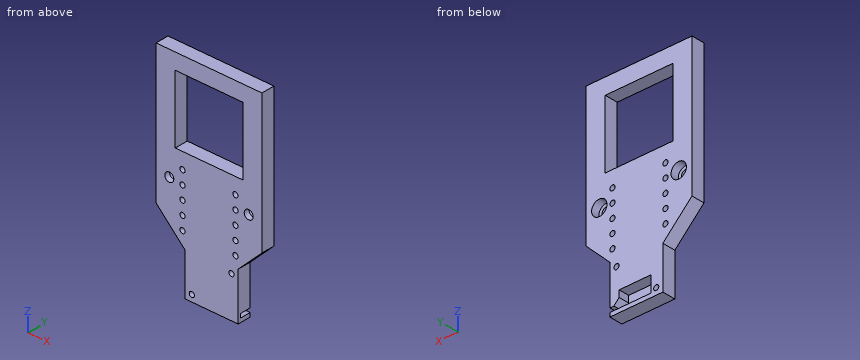
from build123d import *

# Parameters (mm, degrees)
SKETCH1_W           = 40
SKETCH1_H           = 45
SKETCH1_R           = 1.7
BOSS_EXTRUDE1_DEPTH = 5
SKETCH7_R           = 2.9
CUT_EXTRUDE6_DEPTH  = 3
SKETCH4_R           = 0.975
CUT_EXTRUDE3_DEPTH  = 31.516389039
SKETCH5_R           = 0.975
CUT_EXTRUDE4_DEPTH  = 31.516389039
LPATTERN1_COUNT     = 5
LPATTERN1_PITCH     = 5
CUT_EXTRUDE7_DEPTH  = 4
FILLET2_R           = 3
CHAMFER2_SIZE       = 2
CUT_EXTRUDE8_DEPTH  = 31.516389039
SKETCH10_W          = 40
SKETCH10_H          = 34.5
SKETCH10_W_2        = 25.5
SKETCH10_H_2        = 25.5
BOSS_EXTRUDE2_DEPTH = 5


with BuildPart() as part:
    # Sketch1 → Boss-Extrude1 (new body)
    with BuildSketch(Plane(origin=(0, 0, 0), x_dir=(1, 0, 0), z_dir=(0, 1, 0))):
        Rectangle(SKETCH1_W, SKETCH1_H)
        with Locations(Location((-15, 15, 0), (0, 0, 270))):
            Circle(SKETCH1_R, mode=Mode.SUBTRACT)
        with Locations(Location((-15, -15, 0), (0, 0, 270))):
            Circle(SKETCH1_R, mode=Mode.SUBTRACT)
        with Locations(Location((15, -15, 0), (0, 0, 90))):
            Circle(SKETCH1_R, mode=Mode.SUBTRACT)
        with Locations(Location((15, 15, 0), (0, 0, 90))):
            Circle(SKETCH1_R, mode=Mode.SUBTRACT)
    extrude(amount=BOSS_EXTRUDE1_DEPTH)

    # Sketch7 → Cut-Extrude6 (cut)
    with BuildSketch(Plane(origin=(0, 5, 0), x_dir=(1, 0, 0), z_dir=(0, 1, 0))):
        with Locations(Location((-15, 15, 0), (0, 0, 270))):
            Circle(SKETCH7_R)
        with Locations(Location((15, 15, 0), (0, 0, 270))):
            Circle(SKETCH7_R)
        with Locations(Location((-15, -15, 0), (0, 0, 270))):
            Circle(SKETCH7_R)
        with Locations(Location((15, -15, 0), (0, 0, 270))):
            Circle(SKETCH7_R)
    extrude(amount=-CUT_EXTRUDE6_DEPTH, mode=Mode.SUBTRACT)

    # Sketch4 → Cut-Extrude3 (cut, through all)
    with BuildSketch(Plane(origin=(0, 5, 0), x_dir=(1, 0, 0), z_dir=(0, 1, 0))):
        with Locations(Location((-6.5, 20, 0), (0, 0, 270))):
            Circle(SKETCH4_R)
        with Locations(Location((8.5, 7, 0), (0, 0, 270))):
            Circle(SKETCH4_R)
    extrude(amount=-CUT_EXTRUDE3_DEPTH, mode=Mode.SUBTRACT)

    # Sketch5 → Cut-Extrude4 (cut, through all)
    with BuildSketch(Plane(origin=(0, 5, 0), x_dir=(1, 0, 0), z_dir=(0, 1, 0))):
        with Locations(Location((-10, -19.5, 0), (0, 0, 270))):
            Circle(SKETCH5_R)
        with Locations(Location((10, -19.5, 0), (0, 0, 90))):
            Circle(SKETCH5_R)
    cut_extrude4 = extrude(amount=-CUT_EXTRUDE4_DEPTH, mode=Mode.SUBTRACT)

    # LPattern1: Cut-Extrude4 ×5
    with Locations(*[(0, 0, -i * LPATTERN1_PITCH) for i in range(1, LPATTERN1_COUNT)]):
        add(cut_extrude4, mode=Mode.SUBTRACT)

    # Sketch8 → Cut-Extrude7 (cut)
    with BuildSketch(Plane(origin=(0, 5, 0), x_dir=(1, 0, 0), z_dir=(0, 1, 0))):
        Polygon((-4.5, 21), (7.5, 21), (15.5, 21), (15.5, 19.5), (7.5, 19.5), (7.5, 15), (-4.5, 15), align=None)
    extrude(amount=-CUT_EXTRUDE7_DEPTH, mode=Mode.SUBTRACT)

    # Fillet2
    fillet2_edges = [part.edges().sort_by_distance(p)[0] for p in [
        (15.5, 1, -20.25),
    ]]
    fillet(fillet2_edges, radius=FILLET2_R)

    # Chamfer2
    chamfer2_edges = [part.edges().sort_by_distance(p)[0] for p in [
        (7.5, 3, -19.5),
    ]]
    chamfer(chamfer2_edges, length=CHAMFER2_SIZE)

    # Sketch9 → Cut-Extrude8 (cut, through all)
    with BuildSketch(Plane(origin=(0, 5, 0), x_dir=(1, 0, 0), z_dir=(0, 1, 0))):
        Polygon((-9, 22.5), (-9, 6.5), (-20, -4.5), (-20, 22.5), align=None)
        Polygon((20, 22.5), (11, 22.5), (11, 4.5), (20, -4.5), align=None)
    extrude(amount=-CUT_EXTRUDE8_DEPTH, mode=Mode.SUBTRACT)

    # Sketch10 → Boss-Extrude2 (add)
    with BuildSketch(Plane(origin=(0, 5, 0), x_dir=(1, 0, 0), z_dir=(0, 1, 0))):
        with Locations((0, -39.75)):
            Rectangle(SKETCH10_W, SKETCH10_H)
        with Locations((0, -38.25)):
            Rectangle(SKETCH10_W_2, SKETCH10_H_2, mode=Mode.SUBTRACT)
    extrude(amount=-BOSS_EXTRUDE2_DEPTH)


solid = part.part
CAD build for the part. Positions are in the model's coordinates, mm. Round coordinates to 2 decimals unless told otherwise and drop trailing zeros. Order: outer loops, then holes, each group sorted by start corner. A loop starts at its lowest first (then second) coordinate and runs counter-clockwise, first axis right, second up. Notation, with made-up numbers: (-18.5, -28.5) - (35.5, -28.5) arc R23 ccw to (35.5, 7.5) - close; hole circle Ø10 at (31.25, 61.5). An arc over 180 degrees is marked (long way). Return JSON: item names as keys, results as strings.
(1) Pin check, flat tips, straight feed: pin 1 Ø4.5 at (x, z) = (15, 15) entering from +Y; pin 2 Ø1.2 at (y, z) = (3, -17) entering from +X. Stop position of each tip, or through.
Answer key:
{"pin 1": "stops at y = 2", "pin 2": "stops at x = 11"}
(2) Cut at B-B (z = 9.5). Give the cut face in (x, y) (3 decimals), then the cut area to 4 significant figures.
Answer key:
{"outline": "(-20, 0) - (-10.975, 0) - (-10.975, 5) - (-20, 5) - close; (-9.025, 0) - (9.025, 0) - (9.025, 5) - (-9.025, 5) - close; (10.975, 0) - (20, 0) - (20, 5) - (10.975, 5) - close", "area": "180.5 mm^2"}
(3) Cut at A-A (x = 15). Give the cut face in (y, z).
Answer key:
{"outline": "(0, -0.5) - (5, -0.5) - (5, 12.1) - (2, 12.1) - (2, 13.3) - (0, 13.3) - close; (0, 16.7) - (2, 16.7) - (2, 17.9) - (5, 17.9) - (5, 57) - (0, 57) - close"}
(4) Cut at C-C (x = -10). Give the cut face in (y, z) (3 decimals), then the cut area to 3 significant figures.
Answer key:
{"outline": "(0, -5.5) - (5, -5.5) - (5, -1.475) - (0, -1.475) - close; (0, 0.475) - (5, 0.475) - (5, 3.525) - (0, 3.525) - close; (0, 5.475) - (5, 5.475) - (5, 8.525) - (0, 8.525) - close; (0, 10.475) - (5, 10.475) - (5, 13.525) - (0, 13.525) - close; (0, 15.475) - (5, 15.475) - (5, 18.525) - (0, 18.525) - close; (0, 20.475) - (5, 20.475) - (5, 25.5) - (0, 25.5) - close; (0, 51) - (5, 51) - (5, 57) - (0, 57) - close", "area": "136 mm^2"}
(5) Cut at D-D (z = 32). Give the cut face in (x, y), then the cut area to 3 significant figures.
Answer key:
{"outline": "(-20, 0) - (-12.75, 0) - (-12.75, 5) - (-20, 5) - close; (12.75, 0) - (20, 0) - (20, 5) - (12.75, 5) - close", "area": "72.5 mm^2"}
(6) Wall check: probe 1 along Z at (x, y) = (-2, 2.6); probe 2 along X at (y, z) = (1.7, 36); probe 3 along Z at (x, y) = (-8.5, 1.85). Give the ranges that are in metal, low to high. Write a range as from..to.
Answer key:
{"probe 1": "z = -22.5..-21, -15..25.5, 51..57", "probe 2": "x = -20..-12.75, 12.75..20", "probe 3": "z = -22.5..25.5, 51..57"}
